For this review, take the finished solid that the model builds, in its own axes (mm). Face numbers are marked on the shaded views. Round coordinates to 2 decimals unless told otherwise and drop trailing zeros. Write each loop counter-clockwise with the first axis right and the second up, starting at its lowest first coordinate (ties: lowest second). Pieces come first, ordered by that corner, then holes. Notation, with made-up numbers: (31, 79.25) -> (40, 79.25) arc R16 cw to (40, 106.25) -> close; hole circle Ø5 at (82, 76). An arc over 180 degrees is marked (long way). Write item = value, one per line. Start each with the question number.
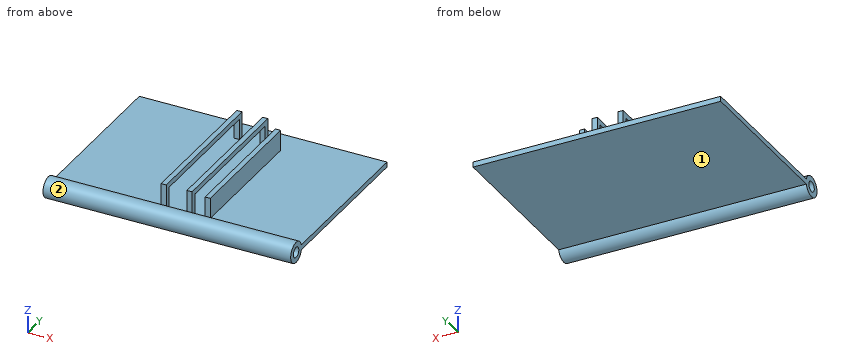
```python
from build123d import *

# Parameters (mm, degrees)
F0_W      = 152.4
F0_H      = 101.6
F1_DEPTH  = 3.175
F2_R      = 6.35
F3_DEPTH  = 76.2
F4_DEPTH  = 76.2
F5_R      = 3.175
F6_DEPTH  = 152.4
F10_DEPTH = 3.175
F13_DEPTH = 3.175
F16_DEPTH = 3.175


# Not quite as in the source:
# - a feature names something its author has since deleted; it is built from what else it names


with BuildPart() as f1:
    # F0 (on Top) → F1 (new body)
    with BuildSketch(Plane.XY):
        Rectangle(F0_W, F0_H)
    extrude(amount=F1_DEPTH)

    # F2 (on Right) → F3 (join)
    with BuildSketch(Plane.YZ):
        with Locations((-55.88, 1.5875)):
            Circle(F2_R)
    extrude(amount=F3_DEPTH)

    # F4 (add): a face of the model
    f4_faces = [f1.faces().sort_by_distance(p)[0] for p in [
        (0, -56.0567159254, 1.5875),
    ]]
    extrude(f4_faces, amount=F4_DEPTH)

    # F5 (on face) → F6 (cut)
    with BuildSketch(Plane.YZ.offset(76.2)):
        with Locations((-55.88, 1.5875)):
            Circle(F5_R)
    extrude(amount=-F6_DEPTH, mode=Mode.SUBTRACT)

    # F9 (on offset) → F10 (join)
    with BuildSketch(Plane.YZ.offset(6.35)):
        Polygon((-50.8, 3.175), (-47.625, 3.175), (-47.625, 15.875), (34.925, 15.875), (34.925, 3.175), (38.1, 3.175), (38.1, 19.05), (-50.8, 19.05), align=None)
    extrude(amount=F10_DEPTH)

    # F12 (on offset) → F13 (join)
    with BuildSketch(Plane.YZ.offset(-6.35)):
        Polygon((-50.8, 3.175), (-47.625, 3.175), (-47.625, 15.875), (34.925, 15.875), (34.925, 3.175), (38.1, 3.175), (38.1, 19.05), (-50.8, 19.05), align=None)
    extrude(amount=-F13_DEPTH)

    # F15 (on offset) → F16 (join)
    with BuildSketch(Plane.YZ.offset(15.875)):
        Polygon((-47.625, 15.875), (-47.625, 3.175), (-47.3777212979, 3.175), (34.925, 3.175), (34.925, 15.875), align=None)
    extrude(amount=F16_DEPTH)


solid = f1.part
```
1. Consider section D-D, the plane y = 42. Give the boundary of the cut face in (x, z) (3 decimals).
2. Draft analysis for pull direction Z (two halves, no side actions). For the marked faces 1 and 2, state which applies: +Z half, -Z half, draft (parallel to the pull), parting line (faces both ways), or undercut.
3. Clearance check with flat-ended pins moving along their axes: pin 1 Ø2.5 at (x, y) = (17.5, -9) entering from +Z (3 decimals); pin 2 Ø6 at (x, y) = (28.5, -25) entering from -Z; pin 3 Ø12.5 at (y, z) = (-28.5, 14.5) entering from +X. State where each tip first meets the part, or that it passes through.
4. Consider section A-A, the plane y = -39. Give the boundary of the cut face in (x, z) (3 decimals).
5. Consider section B-B, the plane y = -55.88. Give the boundary of the cut face in (x, z), then the cut area to 3 significant figures.
6. Wall thickness on L1, parallel to X at y = 8.5, z = 16.25 (3 decimals); L2, parallel to Z at x = 29.5, y = -55.88; L3, parallel to Y at x = 6.5, z = 8.75 (3 decimals): over which ranges is each line inside the solid? List them lowest first. Write a range as from..to.
Outcome:
q1.outline = (-76.2, 0) -> (76.2, 0) -> (76.2, 3.175) -> (-76.2, 3.175) -> close
q2.face_1 = -Z half
q2.face_2 = parting line
q3.pin_1 = 15.875
q3.pin_2 = 0
q3.pin_3 = 19.05
q4.outline = (-76.2, 0) -> (76.2, 0) -> (76.2, 3.175) -> (19.05, 3.175) -> (19.05, 15.875) -> (15.875, 15.875) -> (15.875, 3.175) -> (-76.2, 3.175) -> close; (-9.525, 15.875) -> (-6.35, 15.875) -> (-6.35, 19.05) -> (-9.525, 19.05) -> close; (6.35, 15.875) -> (9.525, 15.875) -> (9.525, 19.05) -> (6.35, 19.05) -> close
q5.outline = (-76.2, -4.76) -> (76.2, -4.76) -> (76.2, -1.59) -> (-76.2, -1.59) -> close; (-76.2, 4.76) -> (76.2, 4.76) -> (76.2, 7.94) -> (-76.2, 7.94) -> close
q5.area = 968 mm2
q6.L1 = -9.525..-6.35, 6.35..9.525
q6.L2 = -4.76..-1.59, 4.76..7.94
q6.L3 = -50.8..-47.625, 34.925..38.1
